The listing builds one solid part. Answer for the finished solid, in the listing's coordinates (mm). A direction names the side the tool comes from. Coordinates: 2 decimals unless noted, no trailing zeros. Write each loop counter-clockwise with the first axis right and the second up, starting at its lowest first coordinate (ties: lowest second). Pieces come first, ordered by that corner, then holes.
from build123d import *

# Parameters (mm, degrees)
SKETCH1_R           = 1.05
BOSS_EXTRUDE1_DEPTH = 1.5
FILLET1_R           = 1.5
SKETCH2_R           = 1.05
SKETCH2_W           = 4
SKETCH2_H           = 16
BOSS_EXTRUDE2_DEPTH = 1.5
SKETCH4_R           = 1.25
CUT_EXTRUDE2_DEPTH  = 160.067595694
CUT_EXTRUDE4_DEPTH  = 160.067595694
FILLET3_R           = 1
CUT_EXTRUDE5_DEPTH  = 160.067595694
BOSS_EXTRUDE3_DEPTH = 1.5
FILLET4_R           = 1.5


with BuildPart() as part:
    # Sketch1 → Boss-Extrude1 (new body)
    with BuildSketch(Plane(origin=(0, 0, 0), x_dir=(0, 0, -1), z_dir=(1, 0, 0))):
        Polygon((0, 0), (0, 75.5), (21.5, 75.5), (40, 0), (35.881667859, 0), (29.755840045, 25), (4, 25), (4, 0), align=None)
        with Locations((5.5, 72.5)):
            Circle(SKETCH1_R, mode=Mode.SUBTRACT)
        with Locations((18.5, 72.5)):
            Circle(SKETCH1_R, mode=Mode.SUBTRACT)
        Polygon((4, 69.5), (18.851866535, 69.5), (4, 29), align=None, mode=Mode.SUBTRACT)
        Polygon((8.260475549, 29), (20.558388216, 62.535546651), (28.775707595, 29), align=None, mode=Mode.SUBTRACT)
    extrude(amount=BOSS_EXTRUDE1_DEPTH)

    # Fillet1
    fillet1_edges = [part.edges().sort_by_distance(p)[0] for p in [
        (0.75, 75.5, -21.5),
        (0.75, 25, -29.755840045),
        (0.75, 25, -4),
        (0.75, 69.5, -4),
        (0.75, 29, -4),
        (0.75, 69.5, -18.851866535),
        (0.75, 29, -8.260475549),
        (0.75, 29, -28.775707595),
        (0.75, 62.535546651, -20.558388216),
    ]]
    fillet(fillet1_edges, radius=FILLET1_R)

    # Sketch2 → Boss-Extrude2 (add)
    # profile 1 of 5: a face of its own
    with BuildSketch(Plane(origin=(1.5, 0, 0), x_dir=(0, 0, -1), z_dir=(1, 0, 0))):
        Polygon((70, 0), (70, 16), (36.079470199, 16), (40, 0), align=None)
    # profile 2 of 5: a face of its own
    with BuildSketch(Plane(origin=(1.5, 0, 0), x_dir=(0, 0, -1), z_dir=(1, 0, 0))):
        with BuildLine():
            Line((103.920529801, 16), (70, 16))
            Line((70, 16), (70, 0))
            Line((70, 0), (140, 0))
            Line((140, 0), (140, 16))
            Line((140, 16), (140, 75.5))
            Line((140, 75.5), (119.676824884, 75.5))
            ThreePointArc((119.676824884, 75.5), (118.750942408, 75.180144754), (118.219924421, 74.356988855))
            Line((118.219924421, 74.356988855), (103.920529801, 16))
        make_face()
        with BuildLine():
            Line((108.038861942, 16), (109.964084377, 23.856988855))
            ThreePointArc((109.964084377, 23.856988855), (110.495102363, 24.680144754), (111.420984839, 25))
            Line((111.420984839, 25), (134.5, 25))
            ThreePointArc((134.5, 25), (135.560660172, 24.560660172), (136, 23.5))
            Line((136, 23.5), (136, 16))
            Line((136, 16), (108.038861942, 16))
        make_face(mode=Mode.SUBTRACT)
        with BuildLine():
            ThreePointArc((131.000070484, 31.016439186), (130.821545012, 29.641122471), (129.591776989, 29))
            Line((129.591776989, 29), (113.136216627, 29))
            ThreePointArc((113.136216627, 29), (111.956071873, 29.574117524), (111.679316165, 30.856988855))
            Line((111.679316165, 30.856988855), (118.270545293, 57.756329353))
            ThreePointArc((118.270545293, 57.756329353), (119.644098522, 58.897023121), (121.135739251, 57.915779684))
            Line((121.135739251, 57.915779684), (131.000070484, 31.016439186))
        make_face(mode=Mode.SUBTRACT)
        with BuildLine():
            ThreePointArc((121.887587432, 67.483560814), (122.066112904, 68.858877529), (123.295880927, 69.5))
            Line((123.295880927, 69.5), (134.5, 69.5))
            ThreePointArc((134.5, 69.5), (135.560660172, 69.060660172), (136, 68))
            Line((136, 68), (136, 37.447151885))
            ThreePointArc((136, 37.447151885), (134.762259183, 35.970256452), (133.091706505, 36.930712699))
            Line((133.091706505, 36.930712699), (121.887587432, 67.483560814))
        make_face(mode=Mode.SUBTRACT)
        with Locations((121.5, 72.5)):
            Circle(SKETCH2_R, mode=Mode.SUBTRACT)
        with Locations((134.5, 72.5)):
            Circle(SKETCH2_R, mode=Mode.SUBTRACT)
    # profile 3 of 5: a face of its own
    with BuildSketch(Plane(origin=(1.5, 0, 0), x_dir=(0, 0, -1), z_dir=(1, 0, 0))):
        Polygon((35.881667859, 0), (31.961138058, 16), (4, 16), (4, 0), align=None)
    # profile 4 of 5: a face of its own
    with BuildSketch(Plane(origin=(1.5, 0, 0), x_dir=(0, 0, -1), z_dir=(1, 0, 0))):
        Polygon((40, 0), (36.079470199, 16), (31.961138058, 16), (35.881667859, 0), align=None)
    # profile 5 of 5: a face of its own
    with BuildSketch(Plane(origin=(1.5, 0, 0), x_dir=(0, 0, -1), z_dir=(1, 0, 0))):
        with Locations((2, 8)):
            Rectangle(SKETCH2_W, SKETCH2_H)
    extrude(amount=-BOSS_EXTRUDE2_DEPTH)

    # Sketch4 → Cut-Extrude2 (cut, through all)
    with BuildSketch(Plane(origin=(1.5, 0, 0), x_dir=(0, 0, -1), z_dir=(1, 0, 0))):
        with Locations((6.1, 8)):
            Circle(SKETCH4_R)
        with Locations((17.1, 8)):
            Circle(SKETCH4_R)
        with Locations(Location((122.9, 8, 0), (0, 0, 180))):
            Circle(SKETCH4_R)
        with Locations(Location((133.9, 8, 0), (0, 0, 180))):
            Circle(SKETCH4_R)
        with BuildLine():
            Line((130.4, 16), (130.4, 8))
            ThreePointArc((130.4, 8), (128.4, 6), (126.4, 8))
            Line((126.4, 8), (126.4, 16))
            Line((126.4, 16), (130.4, 16))
        make_face()
        with BuildLine():
            Line((13.6, 16), (13.6, 8))
            ThreePointArc((13.6, 8), (11.6, 6), (9.6, 8))
            Line((9.6, 8), (9.6, 16))
            Line((9.6, 16), (13.6, 16))
        make_face()
    extrude(amount=-CUT_EXTRUDE2_DEPTH, mode=Mode.SUBTRACT)

    # Sketch5 → Cut-Extrude4 (cut, through all)
    with BuildSketch(Plane(origin=(1.5, 0, 0), x_dir=(0, 0, -1), z_dir=(1, 0, 0))):
        Polygon((35.984634856, 4.5), (46, 4.5), (56.015365144, 4.5), (46, 10.342296334), align=None)
        Polygon((47.984634856, 11.5), (68.015365144, 11.5), (58, 5.657703666), align=None)
        Polygon((59.984634856, 4.5), (70, 4.5), (80.015365144, 4.5), (70, 10.342296334), align=None)
        Polygon((22, 4.5), (22, 10.342296334), (32.015365144, 4.5), align=None)
        Polygon((23.984634856, 11.5), (44.015365144, 11.5), (34, 5.657703666), align=None)
        Polygon((118, 4.5), (118, 10.342296334), (107.984634856, 4.5), align=None)
        Polygon((94, 4.5), (104.015365144, 4.5), (94, 10.342296334), (83.984634856, 4.5), align=None)
        Polygon((95.984634856, 11.5), (116.015365144, 11.5), (106, 5.657703666), align=None)
        Polygon((71.984634856, 11.5), (92.015365144, 11.5), (82, 5.657703666), align=None)
    extrude(amount=-CUT_EXTRUDE4_DEPTH, mode=Mode.SUBTRACT)

    # Fillet3
    fillet3_edges = [part.edges().sort_by_distance(p)[0] for p in [
        (0.75, 4.5, -83.984634856),
        (0.75, 4.5, -104.015365144),
        (0.75, 4.5, -80.015365144),
        (0.75, 4.5, -59.984634856),
        (0.75, 10.342296334, -70),
        (0.75, 4.5, -56.015365144),
        (0.75, 4.5, -35.984634856),
        (0.75, 10.342296334, -46),
        (0.75, 4.5, -118),
        (0.75, 4.5, -107.984634856),
        (0.75, 10.342296334, -118),
        (0.75, 11.5, -44.015365144),
        (0.75, 5.657703666, -34),
        (0.75, 11.5, -23.984634856),
        (0.75, 5.657703666, -58),
        (0.75, 11.5, -47.984634856),
        (0.75, 11.5, -68.015365144),
        (0.75, 11.5, -116.015365144),
        (0.75, 5.657703666, -106),
        (0.75, 11.5, -95.984634856),
        (0.75, 11.5, -92.015365144),
        (0.75, 5.657703666, -82),
        (0.75, 11.5, -71.984634856),
        (0.75, 4.5, -32.015365144),
        (0.75, 4.5, -22),
        (0.75, 10.342296334, -22),
    ]]
    fillet(fillet3_edges, radius=FILLET3_R)

    # Sketch6 → Cut-Extrude5 (cut, through all)
    with BuildSketch(Plane(origin=(1.5, 0, 0), x_dir=(0, 0, -1), z_dir=(1, 0, 0))):
        Polygon((4, 19.75), (30.998526841, 19.928494428), (18.851866535, 69.5), (4, 69.5), align=None)
        Polygon((136, 69.5), (136, 19.75), (109.001473159, 19.928494428), (121.148133465, 69.5), align=None)
    extrude(amount=-CUT_EXTRUDE5_DEPTH, mode=Mode.SUBTRACT)

    # Sketch7 → Boss-Extrude3 (add)
    with BuildSketch(Plane(origin=(1.5, 0, 0), x_dir=(0, 0, -1), z_dir=(1, 0, 0))):
        Polygon((18.851866535, 69.5), (16.776232149, 69.5), (4, 23.476934928), (4, 16), (6.075634386, 16), (19.825004849, 65.528543637), align=None)
        Polygon((136, 16), (136, 23.476934928), (123.223767851, 69.5), (121.148133465, 69.5), (120.174995151, 65.528543637), (133.924365614, 16), align=None)
    extrude(amount=-BOSS_EXTRUDE3_DEPTH)

    # Fillet4
    fillet4_edges = [part.edges().sort_by_distance(p)[0] for p in [
        (0.75, 16, -31.961138058),
        (0.75, 16, -36.079470199),
        (0.75, 16, -108.038861942),
        (0.75, 16, -103.920529801),
        (0.75, 69.5, -4),
        (0.75, 69.5, -136),
        (0.75, 69.5, -16.776232149),
        (0.75, 23.476934928, -4),
        (0.75, 16, -6.075634386),
        (0.75, 65.528543637, -19.825004849),
        (0.75, 23.476934928, -136),
        (0.75, 69.5, -123.223767851),
        (0.75, 65.528543637, -120.174995151),
        (0.75, 16, -133.924365614),
    ]]
    fillet(fillet4_edges, radius=FILLET4_R)


solid = part.part
1. Section D-D on z = -128.4 is taken. Give the vertices of the cut face in (x, y).
Results found:
outline: (0, 0) - (1.5, 0) - (1.5, 6) - (0, 6) - close; (0, 35.9) - (1.5, 35.9) - (1.5, 50.85) - (0, 50.85) - close; (0, 69.5) - (1.5, 69.5) - (1.5, 75.5) - (0, 75.5) - close
2. A tool of negligible diameter and unlimited length cuts with its end or side. For faces 1 (the flat face through (0.76, 7.94, -26.12)), 2 (the flat face through (0.74, 46.15, -28.69)), from which of +Z, -Z, +X, -X, +Y, -Y can it reach the whole face along a straight path? Write none if from no direction.
Results found:
face 1: +X, -X
face 2: +X, -X, +Y
3. Section B-B on z = -72 is taken. Give the vertices of the cut face in (x, y).
Results found:
outline: (0, 0) - (1.5, 0) - (1.5, 4.5) - (0, 4.5) - close; (0, 9.18) - (1.5, 9.18) - (1.5, 16) - (0, 16) - close
4. For a pull along Z with two mould halves and no side action, classify faces 3 (the cylindrical face through (0.76, 8.479, -132.745)), 4 (the flat face through (0, 13, -64)) as pulls with the +Z half, pulls with the -Z half, needs draft (parallel to the pull), parting line crosses it, or undercut.
Results found:
face 3: undercut
face 4: needs draft
5. Find the intervals of material crossed by L1, parallel to Z at x = 0.55, y = 15; L2, parallel to Z at x = 1.1, y = 72.5; L3, parallel to Y at x = 1.3, z = -39.5, in increasing order.
Results found:
L1: z = -140 to -130.4, -126.4 to -13.6, -9.6 to 0
L2: z = -140 to -135.55, -133.45 to -122.55, -120.45 to -117.76, -22.24 to -19.55, -17.45 to -6.55, -4.45 to 0
L3: y = 0 to 4.52, 6.55 to 8.87, 11.5 to 16
6. Flat-ended cylindrical pins translate along their axes: P1, Ø12, axis at y = 11, z = -60, coming from the -X side; P2, Ø2, axis at y = 8, z = -17.1, coming from the +X side. Find the tip coordinate at first contact, or state that the pin passes through.
Results found:
P1: stops at x = 0
P2: passes through
7. Section A-A on y = 14.5 is taken. Give the vertices of the cut face in (x, z).
Results found:
outline: (0, -140) - (1.5, -140) - (1.5, -130.4) - (0, -130.4) - close; (0, -126.4) - (1.5, -126.4) - (1.5, -13.6) - (0, -13.6) - close; (0, -9.6) - (1.5, -9.6) - (1.5, 0) - (0, 0) - close
8. Section C-C on y = 37 is taken. Give the vertices of the cut face in (x, z), then the cut area to 3 significant figures.
Results found:
outline: (0, -140) - (1.5, -140) - (1.5, -136) - (0, -136) - close; (0, -132.25) - (1.5, -132.25) - (1.5, -128.09) - (0, -128.09) - close; (0, -113.18) - (1.5, -113.18) - (1.5, -109.07) - (0, -109.07) - close; (0, -30.93) - (1.5, -30.93) - (1.5, -26.82) - (0, -26.82) - close; (0, -11.91) - (1.5, -11.91) - (1.5, -7.75) - (0, -7.75) - close; (0, -4) - (1.5, -4) - (1.5, 0) - (0, 0) - close
area: 36.8 mm2
